Verification items for this drawing (mm, ordinates from the low corner). A direction names the side the tool comes from. Round coordinates to 2 decimals unless told otherwise and drop trailing zeros. Order: outer loops, then holes, each group sorted by start corner. A loop starts at its lowest first (then second) coordinate and runs counter-clockwise, first axis right, second up. Notation, with made-up numbers: (10, 25) -> (42, 25) arc R29 ccw to (42, 48) -> close; hole circle Ø3 at (88.25, 30). An arc over 180 degrees is marked (long way). Use a Markdown table: item, result. Add a question column.
Item 1: Sectioned sample at C-C, the plane x = 25.75. Record the cut outline in (y, z).
Item 2: Sectioned sample at A-A, the plane z = 4.5. Record the cut outline in (x, y), and give its area (3 significant figures).
Item 3: Material ranges on probe 1 along X at (y, z) = (4, 10); probe 2 along Z at (x, y) = (23.5, 12.5); probe 3 along Y at (x, z) = (21.25, 12.25), recorded low to high. Write a range as [from, to].
Item 4: Gauge pin test, flat ends, axial feed: pin 1 Ø8 at (x, z) = (20, 21) entering from -Y; pin 2 Ø1.5 at (x, z) = (9, 15) entering from -Y; pin 3 Ø6 at (x, z) = (14, 14.5) entering from +Y; pin 4 Ø9 at (y, z) = (12.5, 15) entering from +X. Record the tip position at first contact, or that the pin passes through.
Item 5: Sectioned sample at D-D, the plane y = 12.5. Record the cut outline in (x, z), and give its area (3 significant figures).
Item 6: Mould release check, pull along X, two halves, no side actions. Record for the marked faces 3, 4, 5 and 6: pulls with the +X half, pulls with the -X half, needs draft (parallel to the pull), parting line crosses it, or undercut.
Item 7: Sectioned sample at B-B, the plane y = 2.5. Record the cut outline in (x, z), and give its area (3 significant figures).
Item 8: Set-up check for the marked faces 1 and 2: record each of +Z, -Z, +X, -X, +Y, -Y from which the full face is reachable in a straight line by a thin tool's end or side.
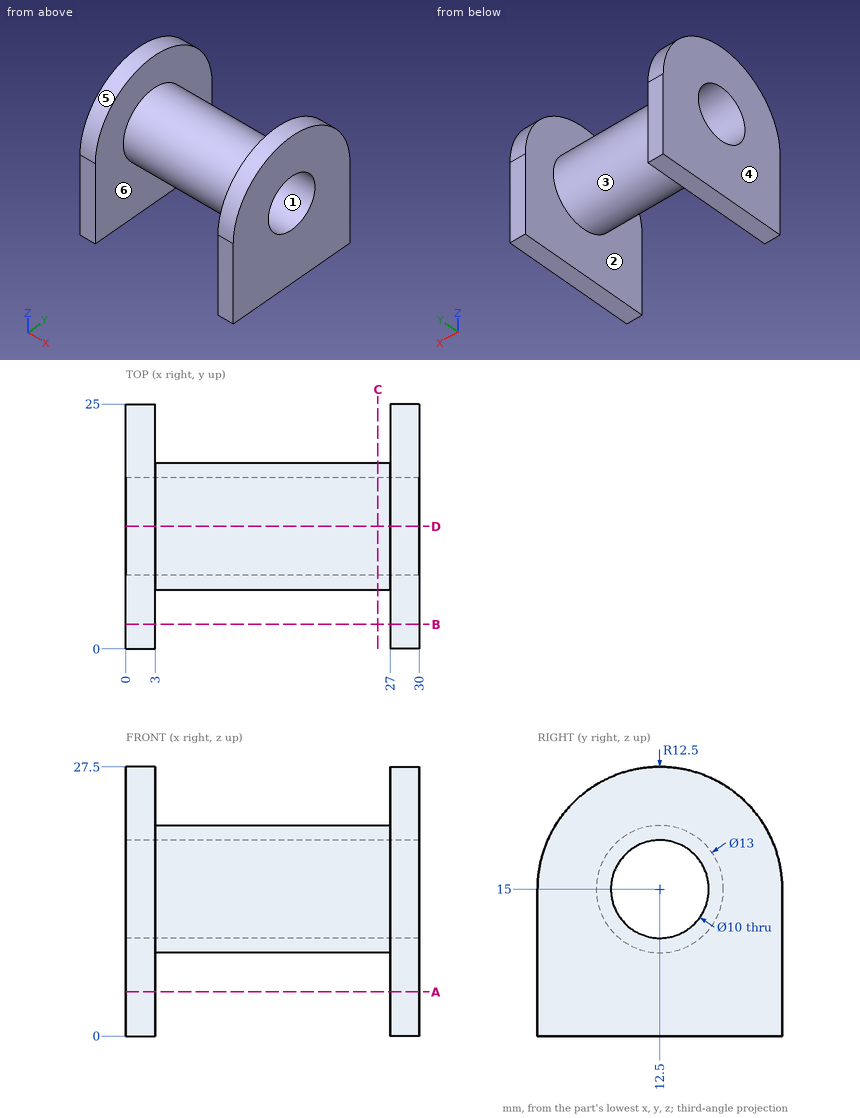
Found:
| question | item | result |
|---|---|---|
| 1 | outline | circle Ø13 at (12.5, 15); hole circle Ø10 at (12.5, 15) |
| 2 | outline | (0, 0) -> (3, 0) -> (3, 25) -> (0, 25) -> close; (27, 0) -> (30, 0) -> (30, 25) -> (27, 25) -> close |
| 2 | area | 150 mm2 |
| 3 | probe 1 | x = [0, 3], [27, 30] |
| 3 | probe 2 | z = [8.5, 10], [20, 21.5] |
| 3 | probe 3 | y = [6.61, 8.32], [16.68, 18.39] |
| 4 | pin 1 | stops at y = 6.32 |
| 4 | pin 2 | stops at y = 6 |
| 4 | pin 3 | stops at y = 19 |
| 4 | pin 4 | passes through |
| 5 | outline | (0, 0) -> (3, 0) -> (3, 8.5) -> (27, 8.5) -> (27, 0) -> (30, 0) -> (30, 10) -> (0, 10) -> close; (0, 20) -> (30, 20) -> (30, 27.5) -> (27, 27.5) -> (27, 21.5) -> (3, 21.5) -> (3, 27.5) -> (0, 27.5) -> close |
| 5 | area | 177 mm2 |
| 6 | face 3 | undercut |
| 6 | face 4 | pulls with the -X half |
| 6 | face 5 | needs draft |
| 6 | face 6 | undercut |
| 7 | outline | (0, 0) -> (3, 0) -> (3, 22.5) -> (0, 22.5) -> close; (27, 0) -> (30, 0) -> (30, 22.5) -> (27, 22.5) -> close |
| 7 | area | 135 mm2 |
| 8 | face 1 | +X, -X |
| 8 | face 2 | none |
